Autodesk Inventor part; units mm, degrees
ref_plane "YZ Plane" through (0, 0, 0) normal (1, 0, 0) x (0, 1, 0)
ref_plane "XZ Plane" through (0, 0, 0) normal (0, 1, 0) x (-1, 0, 0)
ref_plane "XY Plane" through (0, 0, 0) normal (0, 0, 1) x (1, 0, 0)
sketch "스케치1" plane through (0, 0, 0) normal (0, 0, 1) x (1, 0, 0)
  line L0 (-29.5, 14.5) -> (29.5, 14.5)
  line L1 (29.5, 14.5) -> (29.5, -14.5)
  line L2 (29.5, -14.5) -> (-29.5, -14.5)
  line L3 (-29.5, -14.5) -> (-29.5, 14.5)
  line L4 (-29.5, 14.5) -> (29.5, -14.5) construction
  line L5 (29.5, 14.5) -> (-29.5, -14.5) construction
  line L6 (30.5, 15.5) -> (-30.5, 15.5)
  line L7 (-30.5, 15.5) -> (-30.5, -15.5)
  line L8 (-30.5, -15.5) -> (30.5, -15.5)
  line L9 (30.5, -15.5) -> (30.5, 15.5)
  point P0 (0, 0)
  dimension "d0" = 59
  dimension "d1" = 29
  dimension "d4" = 1
extrude "돌출1" add sketch "스케치1" along normal blind 1 contours L0 L1 L2 L3 | L9 L8 L7 L6
sketch "스케치2" plane through (0, 0, 1) normal (0, 0, 1) x (1, 0, 0)
  line L0 (30.5, -15.5) -> (30.5, 15.5)
  line L1 (-30.5, -15.5) -> (30.5, -15.5)
  line L2 (30.5, -15.5) -> (30.5, 15.5)
  line L3 (30.5, 15.5) -> (-30.5, 15.5)
  line L4 (-30.5, 15.5) -> (-30.5, -15.5)
  line L5 (-30.5, -15.5) -> (30.5, 15.5) construction
  line L6 (30.5, -15.5) -> (-30.5, 15.5) construction
  line L7 (-29.5, 14.5) -> (29.5, 14.5)
  line L8 (29.5, 14.5) -> (29.5, -14.5)
  line L9 (29.5, -14.5) -> (-29.5, -14.5)
  line L10 (-29.5, -14.5) -> (-29.5, 14.5)
  point P0 (2.95, 1.45)
  dimension "d5" = 1
extrude "돌출2" add sketch "스케치2" along normal blind 12
sketch "스케치3" plane through (0, 0, 1) normal (0, 0, 1) x (1, 0, 0)
  line L0 (-12.5, -7.5) -> (12.5, -7.5)
  line L1 (12.5, -7.5) -> (12.5, 7.5)
  line L2 (12.5, 7.5) -> (-12.5, 7.5)
  line L3 (-12.5, 7.5) -> (-12.5, -7.5)
  line L4 (-12.5, -7.5) -> (12.5, 7.5) construction
  line L5 (12.5, -7.5) -> (-12.5, 7.5) construction
  point P0 (0, 0)
  dimension "d8" = 25
  dimension "d9" = 15
extrude "돌출3" cut sketch "스케치3" against normal blind 12
sketch "스케치4" plane through (-30.5, -15.5, 0) normal (-1, 0, 0) x (0, 0, 1)
  line L0 (1, 30) -> (13, 30)
  line L1 (1, 1) -> (1, 30)
  line L2 (13, 30) -> (1, 30)
  line L3 (1, 30) -> (1, 1)
  line L4 (1, 1) -> (13, 1)
  line L5 (13, 1) -> (13, 30)
  point P0 (0, 15.5)
extrude "돌출4" cut sketch "스케치4" against normal blind 15
sketch "스케치5" plane through (-30.5, -15.5, 0) normal (-1, 0, 0) x (0, 0, 1)
  line L0 (13, 0) -> (13, 31)
  line L1 (13, 31) -> (14.5, 31)
  line L2 (14.5, 31) -> (14.5, 29)
  line L3 (14.5, 29) -> (13, 29)
  line L4 (13, 29) -> (13, 31)
  line L5 (13, 0) -> (14.5, 0)
  line L6 (14.5, 0) -> (14.5, 2)
  line L7 (14.5, 2) -> (13, 2)
  line L8 (13, 2) -> (13, 0)
  point P0 (0, 15.5)
  point P1 (13, 2)
  dimension "d14" = 1.5
  dimension "d15" = 2
  dimension "d16" = 2
extrude "돌출5" add sketch "스케치5" against normal up to surface (61 mm away)
sketch "스케치6" plane through (-30.5, -15.5, 0) normal (0, -1, 0) x (1, 0, 0)
  line L0 (0, 14.5) -> (61, 14.5)
  line L1 (23, -0.5) -> (38, -0.5)
  line L2 (38, -0.5) -> (38, 14.5)
  line L3 (38, 14.5) -> (23, 14.5)
  line L4 (23, 14.5) -> (23, -0.5)
  line L5 (23, -0.5) -> (38, 14.5) construction
  line L6 (38, -0.5) -> (23, 14.5) construction
  point P0 (30.5, 0)
  point P1 (30.5, 7)
  dimension "d19" = 15
extrude "돌출6" add sketch "스케치6" along normal blind 40
sketch "스케치7" plane through (-30.5, -13.5, 14.5) normal (0, 0, 1) x (1, 0, 0)
  line L0 (38, -42) -> (23, -42)
  line L1 (30.5, -42) -> (30.5, -88)
  circle A0 centre (30.5, -88) radius 46
  circle A1 centre (30.5, -88) radius 43
  line L2 (23, -42) -> (23, -42.6155)
  line L3 (38, -2) -> (38, -42)
  line L4 (38, -42) -> (38, -42.6155)
  line L5 (30.5, -88) -> (32.9075, -133.937)
  line L6 (30.5, -88) -> (76.5, -88) construction
  line L7 (30.5, -88) -> (28.8946, -133.972)
  line L8 (28.8946, -133.972) -> (27.8479, -153.9446)
  line L9 (28.8946, -133.972) -> (48.8946, -133.972) construction
  line L10 (32.9075, -133.937) -> (33.9542, -153.9095)
  line L11 (32.9075, -133.937) -> (52.9075, -133.937) construction
  line L12 (33.9542, -153.9095) -> (38.9511, -153.7351)
  line L13 (33.9542, -153.9095) -> (38.9542, -153.9095) construction
  line L14 (38.9511, -153.7351) -> (38.2598, -133.937)
  line L15 (27.8479, -153.9446) -> (29.0856, -153.9446) construction
  line L16 (38.2598, -133.937) -> (38.2391, -133.3443)
  line L17 (27.8479, -153.9446) -> (22.8548, -153.6829)
  line L18 (27.8479, -153.9446) -> (32.8479, -153.9446) construction
  line L19 (22.8548, -153.6829) -> (23.9112, -133.5257)
  point P0 (30.5, 13.5)
  point P1 (27.1993, -133.8814)
  point P2 (32.7504, -130.9411)
  point P3 (28.9993, -130.9738)
  dimension "d22" = 46
  dimension "d23" = 3
  dimension "d24" = 87
  dimension "d25" = 20
  dimension "d26" = 93
  dimension "d27" = 20
  dimension "d28" = 87
  dimension "d29" = 5
  dimension "d30" = 2
  dimension "d31" = 90
  dimension "d42" = 5
  dimension "d43" = 177
  dimension "d44" = 90
extrude "돌출7" add sketch "스케치7" against normal up to surface (15 mm away) contours L4 A0 L0 | A0 L2 L0 | A0 L5 A1 L1 | L1 A1 L7 A0 | A0 L8 L17 L19 | L16 L14 L12 L10 A0
sketch "스케치9" plane through (7.7391, -146.8443, 14.5) normal (0.9994, 0.0349, 0) x (0, 0, -1)
  line L0 (0, -20.2251) -> (0, 2.6915)
  line L1 (0, -8.7668) -> (15, 1.1952)
  line L2 (15, -0.3012) -> (15, 2.6915)
  circle A0 centre (7.5, -3.7858) radius 3.1
  point P0 (14.5, 147.025)
  point P1 (15, -19.971)
  dimension "d39" = 6.2
extrude "돌출9" cut sketch "스케치9" against normal blind 10
sketch "스케치10" plane through (-7.6452, -167.1829, -0.5) normal (-0.9986, 0.0523, 0) x (0, 0, 1)
  line L0 (15, 0) -> (0, 0)
  line L1 (7.5, 0) -> (7.5, 11.7)
  circle A0 centre (7.5, 11.7) radius 3.1
  point P0 (0.5, 167.3539)
  dimension "d45" = 11.7
  dimension "d46" = 6.2
extrude "돌출10" cut sketch "스케치10" against normal up to surface (5 mm away)
properties part number "camera_robotarm2"
Verification items for the finished model (mm, model axes). A direction names the side the tool comes from. Coordinates: 2 decimals unless noted, no trailing zeros. Write each loop counter-clockwise with the first axis right and the second up, starting at its lowest first coordinate (ties: lowest second). Pieces come first, ordered by that corner, then holes. Notation, with made-up numbers: M 13,-29 L 27,-29 A16 cw 27,-12 Z; hole C -27.5,6.25 d8. An arc over 180 degrees is marked long. One line per item, written item: value.
Item 1: Section check C-C, the plane z = 7.25. State how many separate pieces and enclosed holes the cut face has, plus the area to 3 significant figures.
Check sheet entries:
separate pieces: 3
enclosed holes: 0
area: 1,720 mm^2
Item 2: Access from +Z, -Z, +X, -X, +Y, -Y to the whole of each face (thin tool, end or side, straight path). Record for faces 4 (the cylindrical face through (-1.992, -147.872, 6.893)), 5 (the flat face through (7.5, -36, 7)), 6 (the flat face through (0, 11, 0)), 7 (the flat face through (-1, 14.5, 7)).
Check sheet entries:
face 4: none
face 5: +Z, -Z, +X
face 6: -Z, +X, -X, +Y
face 7: -X
Item 3: Section check B-B, the plane x = 0.5. Record the boundary of the cut face in (y, z).
Check sheet entries:
outline: M -58.5,-0.5 L -15.5,-0.5 L -15.5,0 L -7.5,0 L -7.5,1 L -14.5,1 L -14.5,13 L -13.5,13 L -13.5,14.5 L -58.5,14.5 Z; M 7.5,0 L 15.5,0 L 15.5,14.5 L 13.5,14.5 L 13.5,13 L 14.5,13 L 14.5,1 L 7.5,1 Z
Item 4: Mould release check, pull along Y, two halves, no side actions. Record for faces 1 (the flat face through (-30.5, 1.2, 0.8)), 2 (the flat face through (-1, 9, 1)), 3 (the flat face through (0, 15.5, 7)): pulls with the +Y half, pulls with the -Y half, needs draft (parallel to the pull), parting line crosses it, or undercut.
Check sheet entries:
face 1: needs draft
face 2: undercut
face 3: pulls with the +Y half
Item 5: Scan lines: line 1 along X through (y, z) = (-101.5, 11); line 2 along Y through (x, z) = (-14, 3.5); line 3 along Y through (x, z) = (-3.5, 12.5). Record each from-to range of solid material in increasing order.
Check sheet entries:
line 1: x = -46 to -43, 43 to 46
line 2: y = -145.32 to -142.16, -60.84 to -57.68, -15.5 to -14.5, 14.5 to 15.5
line 3: y = -167.4 to -144.36, -58.64 to -14.5, 14.5 to 15.5
Item 6: Gauge pin test, flat ends, axial feed: pin 1 Ø1.5 at (y, z) = (-67.5, 1.5) entering from -X; pin 2 Ø3.5 at (x, z) = (4.5, 6.5) entering from -Y; pin 3 Ø1.2 at (x, z) = (-0.5, 14) entering from -Y. Record the tip position at first contact, or that the pin passes through.
Check sheet entries:
pin 1: stops at x = -31.79
pin 2: stops at y = -167.41
pin 3: stops at y = -58.51
Item 7: Section check A-A, the plane y = -1. Record the boundary of the cut face in (x, z).
Check sheet entries:
outline: M -30.5,0 L -12.5,0 L -12.5,1 L -30.5,1 Z; M 12.5,0 L 30.5,0 L 30.5,13 L 29.5,13 L 29.5,1 L 12.5,1 Z
Item 8: Section check D-D, the plane x = -19. Record the boundary of the cut face in (y, z).
Check sheet entries:
outline: M -143.39,-0.5 L -140.07,-0.5 L -140.07,14.5 L -143.39,14.5 Z; M -62.93,-0.5 L -59.61,-0.5 L -59.61,14.5 L -62.93,14.5 Z; M -15.5,0 L 15.5,0 L 15.5,14.5 L 13.5,14.5 L 13.5,13 L 14.5,13 L 14.5,1 L -14.5,1 L -14.5,13 L -13.5,13 L -13.5,14.5 L -15.5,14.5 Z
